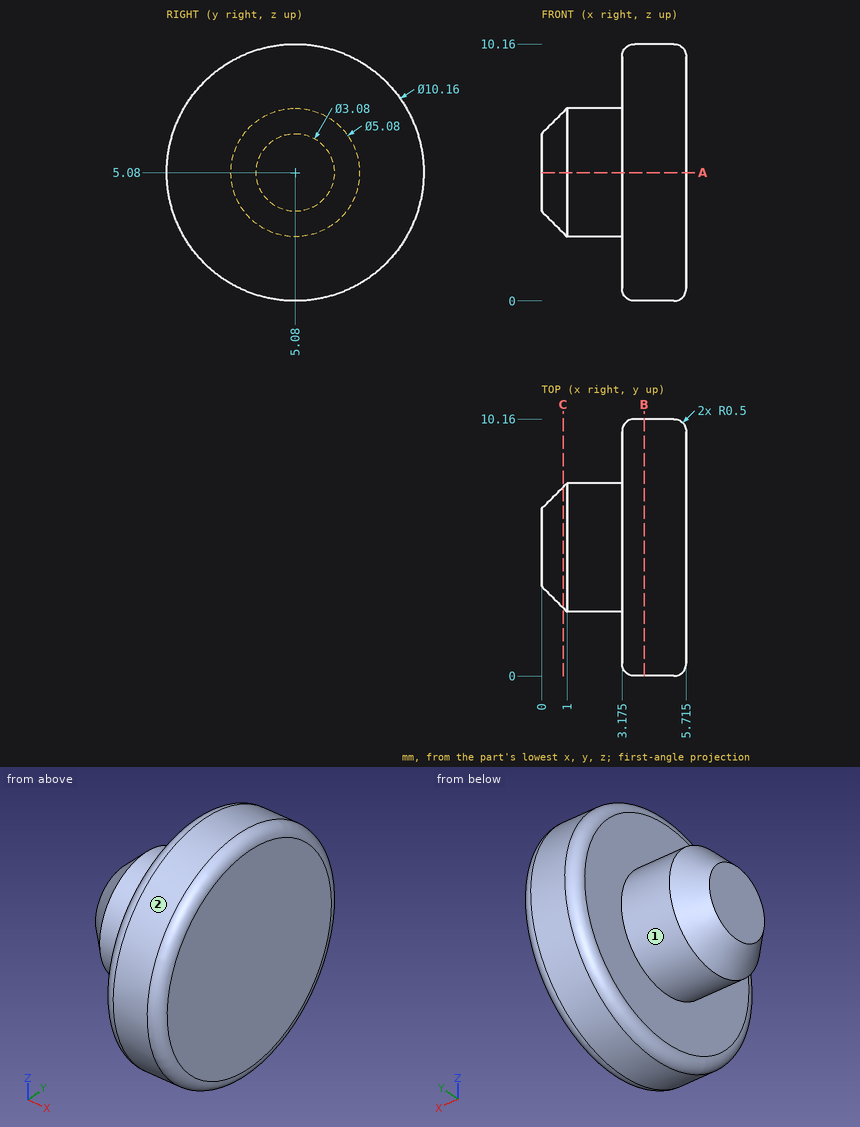
Job drawing, mm, ordinate dimensions from the low corner. One solid piece. A direction names the side the tool comes from. Round coordinates to 2 decimals unless told otherwise and drop trailing zeros. Loops run counter-clockwise (first coordinate to the right, second up) from the corner with the lowest first, then second, coordinate; pieces in that order, holes last. Notation, with made-up numbers: M 71.25,-5.5 L 98.25,-5.5 A24 cw 98.25,24.5 Z; hole C 88.25,12.5 d4. An arc over 180 degrees is marked long. One line per question, with ' | ' between items. Start each with the question number.
Item 1: Pin check, flat tips, straight feed: pin 1 Ø1.5 at (x, z) = (4, 9) entering from +Y; pin 2 Ø1.5 at (x, z) = (4.5, 7) entering from -Y; pin 3 Ø2 at (x, y) = (2.5, 4.5) entering from +Z. Stop position of each tip, or through.
Item 2: Cut at A-A, the plane z = 5.08. Write the cut outline in (x, y) (3 decimals), plus the area to 3 significant figures.
Item 3: Cut at B-B, the plane x = 4.05. Write the cut outline in (y, z).
Item 4: Which spindle directions (+Z, -Z, +X, -X, +Y, -Y) get a long thin tool onto all of the face, cutting with end or side? Do the marked faces 1 and 2. Say none if no direction does.
Item 5: Cut at C-C, the plane x = 0.85. Write the cut outline in (y, z).
Item 6: Wall check: line 1 (X direction, y = 8, z = 3) (3 decimals); line 2 (Z direction, x = 4.4, y = 0.5); line 3 (Z direction, x = 1.4, y = 5). Give the ranges that are in metal, low to high.
Responses:
1) pin 1: stops at y = 9.05 | pin 2: stops at y = 0.14 | pin 3: stops at z = 10.11
2) outline: M 0,3.54 L 1,2.54 L 3.175,2.54 L 3.175,0.5 A0.5 ccw 3.675,0 L 5.215,0 A0.5 ccw 5.715,0.5 L 5.715,9.66 A0.5 ccw 5.215,10.16 L 3.675,10.16 A0.5 ccw 3.175,9.66 L 3.175,7.62 L 1,7.62 L 0,6.62 Z | area: 40.7 mm²
3) outline: C 5.08,5.08 d10.16
4) face 1: -X | face 2: +X, -X
5) outline: C 5.08,5.08 d4.78
6) line 1: x = 3.175 to 5.715 | line 2: z = 2.88 to 7.28 | line 3: z = 2.54 to 7.62
